Can you work these out from the model? Positions are in its coordinate system, mm. Face numbers are marked on the shaded views. A direction names the side the tool comes from. Coordinates: 2 decimals unless noted, no trailing zeros. Order: outer loops, then holes, each group sorted by start corner. A loop starts at its lowest first (then second) coordinate and runs counter-clockwise, first axis right, second up. Notation, with made-up numbers: (68.25, 72.5) -> (82.25, 72.5) arc R17 ccw to (82.25, 99.5) -> close; hole circle Ø3 at (24, -32.75). An arc over 180 degrees is marked (long way). Use a Markdown table: item, result. Add a question column.
1. If I drill on line 1 along X through (y, z) = (-83.5, -39); line 2 along Y through (x, z) = (-10, -22.5); line 3 along Y through (x, z) = (-1, -30), over which ranges is the centre line in solid material (lowest first)? Write a range as from..to.
2. For pin 1 Ø3 at (x, z) = (-17.5, -11.5) entering from -Y, with a flat end and sliding along its axis, tell me the tip position at first contact or that it passes through.
3. Suppose I cut it at C-C, the plane y = -75. List the corners of the cut face in (x, z) for me, then the cut area to 3 significant figures.
4. Suppose I cut it at D-D, the plane x = -18. List the corners of the cut face in (y, z) for me, then the cut area to 3 significant figures.
5. Suppose I cut it at A-A, the plane z = -30. List the corners of the cut face in (x, y) for me.
6. We'd pull the mould along X, two halves only. Please class the marked faces 1, 2 and 3: pulls with the +X half, pulls with the -X half, needs draft (parallel to the pull), parting line crosses it, or undercut.
7. For the marked faces 4 and 5, which set-ups out of +Z, -Z, +X, -X, +Y, -Y let a thin tool reach every point of the face, with its end or its side?
8. Suppose I cut it at B-B, the plane y = -29.5. List the corners of the cut face in (x, z) for me, then the cut area to 3 significant figures.
```python
from build123d import *

# Parameters (mm, degrees)
SKETCH1_R           = 6
BOSS_EXTRUDE1_DEPTH = 3
SKETCH2_W           = 60
SKETCH2_H           = 3
BOSS_EXTRUDE2_DEPTH = 30
SKETCH3_R           = 6
BOSS_EXTRUDE4_DEPTH = 3
FILLET1_R           = 3


with BuildPart() as part:
    # Sketch1 → Boss-Extrude1 (new body)
    with BuildSketch(Plane(origin=(0, 0, 0), x_dir=(0, 0, -1), z_dir=(1, 0, 0))):
        with BuildLine():
            Line((0, 0), (60, 0))
            Line((60, 0), (60, -60))
            ThreePointArc((60, -60), (30, -90), (0, -60))
            Line((0, -60), (0, 0))
        make_face()
        with Locations((30, -75)):
            Circle(SKETCH1_R, mode=Mode.SUBTRACT)
    extrude(amount=-BOSS_EXTRUDE1_DEPTH)

    # Sketch2 → Boss-Extrude2 (add)
    with BuildSketch(Plane.ZY.offset(3)):
        with Locations((-30, -1.5)):
            Rectangle(SKETCH2_W, SKETCH2_H)
    extrude(amount=BOSS_EXTRUDE2_DEPTH)

    # Sketch3 → Boss-Extrude4 (add)
    with BuildSketch(Plane.ZY.offset(33)):
        with BuildLine():
            Line((-60, 0), (0, 0))
            Line((0, 0), (0, -60))
            ThreePointArc((0, -60), (-30, -90), (-60, -60))
            Line((-60, -60), (-60, 0))
        make_face()
        with Locations((-30, -75)):
            Circle(SKETCH3_R, mode=Mode.SUBTRACT)
    extrude(amount=BOSS_EXTRUDE4_DEPTH)

    # Fillet1
    fillet1_edges = [part.edges().sort_by_distance(p)[0] for p in [
        (-36, 0, -30),
        (0, 0, -30),
    ]]
    fillet(fillet1_edges, radius=FILLET1_R)


solid = part.part
```
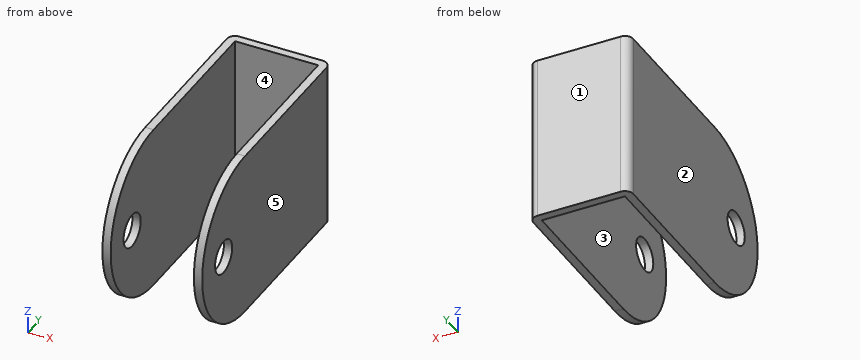
Worked out:
| question | item | result |
|---|---|---|
| 1 | line 1 | x = -36..-33, -3..0 |
| 1 | line 2 | y = -3..0 |
| 1 | line 3 | y = -90..-81, -69..-0.76 |
| 2 | pin 1 | stops at y = -3 |
| 3 | outline | (-36, -55.98) -> (-33, -55.98) -> (-33, -36) -> (-36, -36) -> close; (-36, -24) -> (-33, -24) -> (-33, -4.02) -> (-36, -4.02) -> close; (-3, -55.98) -> (0, -55.98) -> (0, -36) -> (-3, -36) -> close; (-3, -24) -> (0, -24) -> (0, -4.02) -> (-3, -4.02) -> close |
| 3 | area | 240 mm² |
| 4 | outline | (-3, -60) -> (0, -60) -> (0, 0) -> (-3, 0) -> close |
| 4 | area | 180 mm² |
| 5 | outline | (-36, -90) -> (-33, -90) -> (-33, -81) -> (-36, -81) -> close; (-36, -69) -> (-33, -69) -> (-33, -3) -> (-3, -3) -> (-3, -69) -> (0, -69) -> (0, -3) arc R3 ccw to (-3, 0) -> (-33, 0) arc R3 ccw to (-36, -3) -> close; (-3, -90) -> (0, -90) -> (0, -81) -> (-3, -81) -> close |
| 6 | face 1 | needs draft |
| 6 | face 2 | pulls with the -X half |
| 6 | face 3 | undercut |
| 7 | face 4 | +Z, -Z, -Y |
| 7 | face 5 | +Z, -Z, +X, +Y, -Y |
| 8 | outline | (-36, -60) -> (-33, -60) -> (-33, 0) -> (-36, 0) -> close; (-3, -60) -> (0, -60) -> (0, 0) -> (-3, 0) -> close |
| 8 | area | 360 mm² |
